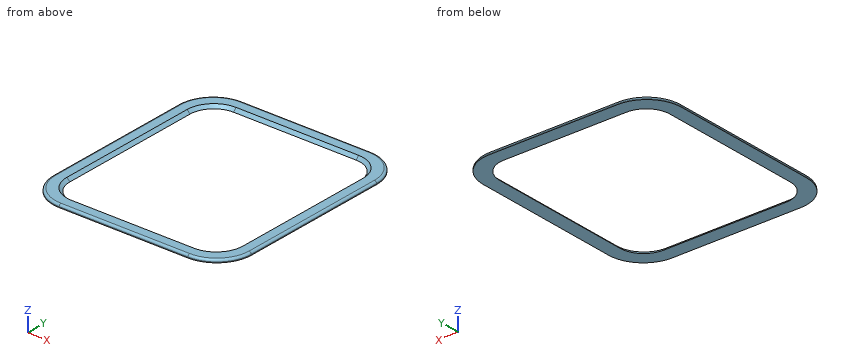
```python
from build123d import *

# Parameters (mm, degrees)
F2_DEPTH     = 1.2065
F3_DEPTH     = 1.2075
F4_R         = 0.8763
F5_T1_DEPTH  = 58.42
F5_T3_DEPTH  = 49.6062
F5_T6_ANGLE  = 90
F5_T8_ANGLE  = 90
F5_T10_ANGLE = 90
F5_T12_ANGLE = 90


# Not quite as in the source:
# - a fillet or chamfer that OpenCascade refuses, or shapes differently, is made with other operations: its cross-section is extruded or revolved along the edge and cut away or added


with BuildPart() as f2:
    # F0 (on Top) → F2 (new body)
    with BuildSketch(Plane.XY):
        with BuildLine():
            ThreePointArc((40.0431, 30.4673), (35.9476619893, 40.3545619893), (26.0604, 44.45))
            Line((26.0604, 44.45), (-26.0604, 44.45))
            ThreePointArc((-26.0604, 44.45), (-35.9476619893, 40.3545619893), (-40.0431, 30.4673))
            Line((-40.0431, 30.4673), (-40.0431, -30.4673))
            ThreePointArc((-40.0431, -30.4673), (-35.9476619893, -40.3545619893), (-26.0604, -44.45))
            Line((-26.0604, -44.45), (26.0604, -44.45))
            ThreePointArc((26.0604, -44.45), (35.9476619893, -40.3545619893), (40.0431, -30.4673))
            Line((40.0431, -30.4673), (40.0431, 30.4673))
        make_face()
    extrude(amount=F2_DEPTH)

    # F1 (on Top) + F2_face (on face) → F3 (cut, through all)
    with BuildSketch(Plane.XY):
        with BuildLine():
            ThreePointArc((34.3281, 29.21), (31.5382920908, 35.9451920908), (24.8031, 38.735))
            Line((24.8031, 38.735), (-24.8031, 38.735))
            ThreePointArc((-24.8031, 38.735), (-31.5382920908, 35.9451920908), (-34.3281, 29.21))
            Line((-34.3281, 29.21), (-34.3281, -29.21))
            ThreePointArc((-34.3281, -29.21), (-31.5382920908, -35.9451920908), (-24.8031, -38.735))
            Line((-24.8031, -38.735), (24.8031, -38.735))
            ThreePointArc((24.8031, -38.735), (31.5382920908, -35.9451920908), (34.3281, -29.21))
            Line((34.3281, -29.21), (34.3281, 29.21))
        make_face()
    with BuildSketch(Plane.XY.offset(1.2065)):
        with BuildLine():
            ThreePointArc((40.0431, 30.4673), (35.9476619893, 40.3545619893), (26.0604, 44.45))
            Line((26.0604, 44.45), (-26.0604, 44.45))
            ThreePointArc((-26.0604, 44.45), (-35.9476619893, 40.3545619893), (-40.0431, 30.4673))
            Line((-40.0431, 30.4673), (-40.0431, -30.4673))
            ThreePointArc((-40.0431, -30.4673), (-35.9476619893, -40.3545619893), (-26.0604, -44.45))
            Line((-26.0604, -44.45), (26.0604, -44.45))
            ThreePointArc((26.0604, -44.45), (35.9476619893, -40.3545619893), (40.0431, -30.4673))
            Line((40.0431, -30.4673), (40.0431, 30.4673))
        make_face()
    extrude(amount=F3_DEPTH, mode=Mode.SUBTRACT)

    # F4
    f4_edges = [f2.edges().sort_by_distance(p)[0] for p in [
        (-40.0431, 0, 1.2065),
    ]]
    fillet(f4_edges, radius=F4_R)

    # F5: chamfer of 1.27 on 1 edges, made by hand

    # F5_s2 → F5_t1 (cut)
    with BuildSketch(Plane.XZ.offset(-29.21)):
        Polygon((-35.5981, 1.2065), (-34.3281, -0.0635), (-34.3281, 1.2065), align=None)
        Polygon((35.5981, 1.2065), (34.3281, -0.0635), (34.3281, 1.2065), align=None)
    extrude(amount=F5_T1_DEPTH, mode=Mode.SUBTRACT)

    # F5_s4 → F5_t3 (cut)
    with BuildSketch(Plane.YZ.offset(-24.8031)):
        Polygon((-40.005, 1.2065), (-38.735, -0.0635), (-38.735, 1.2065), align=None)
        Polygon((40.005, 1.2065), (38.735, -0.0635), (38.735, 1.2065), align=None)
    extrude(amount=F5_T3_DEPTH, mode=Mode.SUBTRACT)

    # F5_s5 → F5_t6 (revolve, cut)
    with BuildSketch(Plane.XZ.offset(-29.21)):
        Polygon((-35.5981, 1.2065), (-34.3281, -0.0635), (-34.3281, 1.2065), align=None)
    revolve(axis=Axis((-24.8031, 29.21, 1.2065), (0, 0, -1)), revolution_arc=F5_T6_ANGLE, mode=Mode.SUBTRACT)

    # F5_s7 → F5_t8 (revolve, cut)
    with BuildSketch(Plane.YZ.offset(-24.8031)):
        Polygon((-40.005, 1.2065), (-38.735, -0.0635), (-38.735, 1.2065), align=None)
    revolve(axis=Axis((-24.8031, -29.21, 1.2065), (0, 0, -1)), revolution_arc=F5_T8_ANGLE, mode=Mode.SUBTRACT)

    # F5_s9 → F5_t10 (revolve, cut)
    with BuildSketch(Plane.XZ.offset(29.21)):
        Polygon((35.5981, 1.2065), (34.3281, -0.0635), (34.3281, 1.2065), align=None)
    revolve(axis=Axis((24.8031, -29.21, 1.2065), (0, 0, -1)), revolution_arc=F5_T10_ANGLE, mode=Mode.SUBTRACT)

    # F5_s11 → F5_t12 (revolve, cut)
    with BuildSketch(Plane.YZ.offset(24.8031)):
        Polygon((40.005, 1.2065), (38.735, -0.0635), (38.735, 1.2065), align=None)
    revolve(axis=Axis((24.8031, 29.21, 1.2065), (0, 0, -1)), revolution_arc=F5_T12_ANGLE, mode=Mode.SUBTRACT)


solid = f2.part
```
CAD build for the part. Positions are in the model's coordinates, mm. Round coordinates to 2 decimals unless told otherwise and drop trailing zeros. Order: outer loops, then holes, each group sorted by start corner. A loop starts at its lowest first (then second) coordinate and runs counter-clockwise, first axis right, second up. Notation, with made-up numbers: (14, -33) - (50, -33) arc R29 ccw to (50, -7) - close; hole circle Ø8 at (-22, -8.75). An arc over 180 degrees is marked (long way). Answer as CSV lines item,"result". Start each with the question number.
1. Saw through at B-B, the plane y = -3.5. Write the cut outline in (x, z).
2. Saw through at C-C, the plane z = 0.7. Write the cut outline in (x, y).
3. Drill centre lines: L1, parallel to Y at x = -7.5, z = 0.35; L2, parallel to X at y = -30, z = 0.45; L3, parallel to Y at x = -10, z = 0.1. Where is each one in solid material? Low to high. Write a range as [from, to].
Model answer:
1,outline,"(-40.04, 0) - (-34.39, 0) - (-35.6, 1.21) - (-39.17, 1.21) arc R0.88 ccw to (-40.04, 0.33) - close; (34.39, 0) - (40.04, 0) - (40.04, 0.33) arc R0.88 ccw to (39.17, 1.21) - (35.6, 1.21) - close"
2,outline,"(-39.96, -30.47) arc R13.9 ccw to (-26.06, -44.37) - (26.06, -44.37) arc R13.9 ccw to (39.96, -30.47) - (39.96, 30.47) arc R13.9 ccw to (26.06, 44.37) - (-26.06, 44.37) arc R13.9 ccw to (-39.96, 30.47) - close; hole (-35.09, -29.21) arc R10.29 ccw to (-24.8, -39.5) - (24.8, -39.5) arc R10.29 ccw to (35.09, -29.21) - (35.09, 29.21) arc R10.29 ccw to (24.8, 39.5) - (-24.8, 39.5) arc R10.29 ccw to (-35.09, 29.21) - close"
3,L1,"y = [-44.45, -39.15], [39.15, 44.45]"
3,L2,"x = [-40.03, -34.81], [34.81, 40.03]"
3,L3,"y = [-44.45, -38.9], [38.9, 44.45]"
